Build history of the part. All positions in model axes, mm. A direction names the side the tool comes from. Coordinates: 2 decimals unless noted, no trailing zeros. Loops run counter-clockwise (first coordinate to the right, second up) from the corner with the lowest first, then second, coordinate; pieces in that order, holes last.
Item 1: Cut at A-A (y = -6). List the corners of the cut face in (x, z), and give its area (3 significant figures).
Item 2: Cut at D-D (x = -8.75). List the corners of the cut face in (y, z), and give its area (3 significant figures).
Item 3: Cut at C-C (x = 1.75). List the corners of the cut face in (y, z).
Item 4: Drill centre lines: line 1 along Y through (x, z) = (0, 15.8); line 2 along X through (y, z) = (8.5, 11); line 3 along Y through (x, z) = (6.75, 7.75). Where is each one in solid material? Low to high.
Item 5: Mould opens along X. For faces 1 (the face through (-3, -1, 11)), 2 (the face through (9.3, -11.8, 0.6)), 3 (the face through (-2.6, -12, 16.5)) say: released by +X, released by -X, zero draft, split by the parting line, or undercut.
Item 6: 3-axis set-ups, long thin cutter, end or side, ignore diameter. For faces 4 (the face through (1.01, -2.45, 8.26)), 5 (the face through (-10, 9.85, 6)): which of +Z, -Z, +X, -X, +Y, -Y reach the whole face in a straight line?
Item 7: Cut at B-B (z = 8). Count the separate pieces of the cut face and the enclosed holes in it, and give its area (3 significant figures).
Item 8: Flat gauge pins, fed straight in: pin 1 (0.7 mm diameter, centred on x = -1, y = -3.5, fed in from -Z); pin 2 (3 mm diameter, centred on x = 1, y = -1, fed in from -Z); pin 3 (3 mm diameter, centred on x = 1.5, y = 1, fed in from -Z). Where does each tip first touch, or does it go through?
Autodesk Inventor part; units mm, degrees
ref_plane "YZ Plane" through (0, 0, 0) normal (1, 0, 0) x (0, 1, 0)
ref_plane "XZ Plane" through (0, 0, 0) normal (0, 1, 0) x (-1, 0, 0)
ref_plane "XY Plane" through (0, 0, 0) normal (0, 0, 1) x (1, 0, 0)
sketch "スケッチ1" plane through (0, 0, 0) normal (0, 0, 1) x (1, 0, 0)
  circle A0 centre (0, 0) radius 5.1
  line L0 (10, -12.5) -> (-10, -12.5)
  line L1 (-10, -12.5) -> (-10, 12.5)
  line L2 (-10, 12.5) -> (10, 12.5)
  line L3 (10, 12.5) -> (10, -12.5)
  line L4 (10, -12.5) -> (-10, 12.5) construction
  line L5 (-10, -12.5) -> (10, 12.5) construction
  dimension "d0" = 10.2
  dimension "d1" = 25
  dimension "d2" = 20
extrude "押し出し1" add sketch "スケッチ1" along normal blind 17
sketch "スケッチ2" plane through (0, 0, 17) normal (0, 0, 1) x (1, 0, 0)
  circle A0 centre (0, 0) radius 5.1
extrude "押し出し2" add sketch "スケッチ2" against normal blind 12
sketch "スケッチ3" plane through (0, 0, 17) normal (0, 0, 1) x (1, 0, 0)
  point P0 (0, 0)
hole "穴1" at (0, 0, 17) direction (0, 0, -1) diameter 5.3 depth 58 counterbore diameter 11 counterbore depth 6
sketch "Sketch7" plane through (-10, -12.5, 0) normal (-1, 0, 0) x (0, 0, 1)
  line L0 (0, 25) -> (0, 0)
  line L1 (5, 7.4) -> (5, 17.6)
  line L2 (0, 17.6) -> (0, 7.4)
  point P0 (0, 12.5)
  point P1 (8, 6.5)
  point P2 (8, 18.5)
  dimension "d35" = 8
  dimension "d36" = 12
  dimension "d37" = 6
hole "Hole3" at (-10, -6, 8) at (-10, 6, 8) direction (1, 0, 0) diameter 4.5 depth 58
chamfer "Chamfer2" distance 3 angle 45 1 edges at (10, 0, 17)
sketch "Sketch8" plane through (-10, -12.5, 0) normal (-1, 0, 0) x (0, 0, 1)
  circle A0 centre (8, 6.5) radius 2.25
  circle A1 centre (8, 18.5) radius 2.25
  line L0 (0, 25) -> (0, 0)
  line L1 (0, 0) -> (17, 0)
  line L2 (17, 25) -> (17, 0)
  line L3 (0, 25) -> (17, 25)
  point P0 (0, 12.5)
extrude "Extrusion5" add sketch "Sketch8" along normal blind 5
sketch "Sketch9" plane through (0, 0, 17) normal (0, 0, 1) x (1, 0, 0)
  line L0 (7, 12.5) -> (7, -12.5)
  line L1 (7, 12.5) -> (-15, 12.5)
  line L2 (-15, -12.5) -> (-15, 12.5)
  line L3 (7, -12.5) -> (-15, -12.5)
  circle A0 centre (0, 0) radius 5.5
  line L4 (-15, 3.75) -> (-15, 8.25)
  line L5 (10, 8.25) -> (10, 3.75)
  line L6 (-15, -8.25) -> (-15, -3.75)
  line L7 (-15, -8.25) -> (-15, -3.75)
  line L8 (10, -3.75) -> (10, -8.25)
  line L9 (-10.9, 9.85) -> (-9.1, 9.85)
  line L10 (-9.1, 9.85) -> (-9.1, 2.15)
  line L11 (-9.1, 2.15) -> (-10.9, 2.15)
  line L12 (-10.9, 2.15) -> (-10.9, 9.85)
  line L13 (-10.9, 9.85) -> (-9.1, 2.15) construction
  line L14 (-9.1, 9.85) -> (-10.9, 2.15) construction
  line L15 (-10.9, -2.15) -> (-9.1, -2.15)
  line L16 (-9.1, -2.15) -> (-9.1, -9.85)
  line L17 (-9.1, -9.85) -> (-10.9, -9.85)
  line L18 (-10.9, -9.85) -> (-10.9, -2.15)
  line L19 (-10.9, -2.15) -> (-9.1, -9.85) construction
  line L20 (-9.1, -2.15) -> (-10.9, -9.85) construction
  line L21 (10, 8.25) -> (10, 3.75)
  point P0 (-10, 6)
  point P1 (-10, -6)
  point P2 (-10, 6)
  point P3 (-10, -6)
  point P4 (10, 6)
  point P5 (10, -6)
  point P6 (10, 6)
  dimension "d53" = 7.7
  dimension "d54" = 7.7
  dimension "d55" = 1.8
  dimension "d56" = 5
extrude "Extrusion6" cut sketch "Sketch9" against normal through all contours L9 L10 L11 L12 | L15 L16 L17 L18
sketch "Sketch10" plane through (0, 0, 17) normal (0, 0, 1) x (1, 0, 0)
  line L0 (-9.1, -2.15) -> (-9.1, -9.85)
  line L1 (-9.1, -9.85) -> (-10.9, -9.85)
  line L2 (-10.9, -9.85) -> (-10.9, -2.15)
  line L3 (-10.9, -2.15) -> (-9.1, -2.15)
  line L4 (-10.9, 9.85) -> (-9.1, 9.85)
  line L5 (-9.1, 9.85) -> (-9.1, 2.15)
  line L6 (-9.1, 2.15) -> (-10.9, 2.15)
  line L7 (-10.9, 2.15) -> (-10.9, 9.85)
  line L8 (7, 12.5) -> (7, -12.5)
  line L9 (7, 12.5) -> (-15, 12.5)
  line L10 (-15, -12.5) -> (-15, 12.5)
  line L11 (7, -12.5) -> (-15, -12.5)
  circle A0 centre (0, 0) radius 5.5
extrude "Extrusion7" add sketch "Sketch10" against normal blind 5 contours L0 L1 L2 L3 | L4 L5 L6 L7
chamfer "Chamfer4" distance 3 angle 45 1 edges at (-15, 0, 17)
chamfer "面取り7" distance 1 angle 45 14 edges at (-15, 12.5, 7) (-13.5, 12.5, 15.5) (-2.5, 12.5, 17) (8.5, 12.5, 15.5) (10, 12.5, 7) (10, -12.5, 7) (8.5, -12.5, 15.5) (-2.5, -12.5, 17) (-13.5, -12.5, 15.5) (-15, -12.5, 7) (-2.5, 12.5, 0) (-2.5, -12.5, 0) (10, 0, 0) (-15, 0, 0)
sketch "スケッチ11" plane through (0, 0, 5) normal (0, 0, -1) x (-1, 0, 0)
  circle A0 centre (0, 0) radius 2.65
  line L0 (2.65, 2.65) -> (-2.65, 2.65)
  line L1 (-2.65, 2.65) -> (-2.65, -2.65)
  line L2 (-2.65, -2.65) -> (2.65, -2.65)
  line L3 (2.65, -2.65) -> (2.65, 2.65)
  circle A1 centre (0, 0) radius 2.65
  line L4 (2.65, 2.65) -> (-2.65, -2.65) construction
  line L5 (-2.65, 2.65) -> (2.65, -2.65) construction
  point P0 (2.65, 0)
  point P1 (0, -2.65)
  point P2 (0, 2.65)
  point P3 (-2.65, 0)
extrude "押し出し8" cut sketch "スケッチ11" against normal blind 0.6 contours L3 L2 A0 | A0 L0 L3 | A0 L1 L0 | L2 L1 A0
sketch "スケッチ12" plane through (0, 0, 5) normal (0, 0, -1) x (-1, 0, 0)
  line L0 (-2.65, 2.65) -> (2.65, 2.65)
  line L1 (2.65, -2.65) -> (-2.65, -2.65)
  circle A0 centre (0, 0) radius 5.1
  line L2 (2.65, 5.3923) -> (-2.65, 5.3923)
  line L3 (-2.65, 5.3923) -> (-2.65, -5.3923)
  line L4 (-2.65, -5.3923) -> (2.65, -5.3923)
  line L5 (2.65, -5.3923) -> (2.65, 5.3923)
  line L6 (2.65, 5.3923) -> (-2.65, -5.3923) construction
  line L7 (-2.65, 5.3923) -> (2.65, -5.3923) construction
  point P0 (2.65, 2.65)
  point P1 (2.65, 4.3575)
  point P2 (-2.65, 4.3575)
  point P3 (2.65, -4.3575)
  point P4 (-2.65, -4.3575)
extrude "押し出し9" cut sketch "スケッチ12" against normal blind 0.3 contours L3 A0 L5 L0 | L1 L5 A0 L3
properties part number "Print_Parts_R" material "PC/ABS プラスチック"
Filled sheet:
1. outline: (-15, 1) - (-14, 0) - (-10.9, 0) - (-10.9, 5.75) - (-15, 5.75) - close; (-15, 10.25) - (-10.9, 10.25) - (-10.9, 12) - (-9.1, 12) - (-9.1, 10.25) - (10, 10.25) - (10, 14) - (7, 17) - (-12, 17) - (-15, 14) - close; (-9.1, 0) - (9, 0) - (10, 1) - (10, 5.75) - (-9.1, 5.75) - close
1. area: 289 mm2
2. outline: (-12.5, 1) - (-11.5, 0) - (11.5, 0) - (12.5, 1) - (12.5, 16) - (11.5, 17) - (-11.5, 17) - (-12.5, 16) - close; hole circle Ø4.5 at (-6, 8); hole circle Ø4.5 at (6, 8)
2. area: 391 mm2
3. outline: (-12.5, 1) - (-11.5, 0) - (-4.79, 0) - (-4.79, 5.3) - (-2.65, 5.3) - (-2.65, 5.6) - (-1.99, 5.6) - (-1.99, 11) - (-5.21, 11) - (-5.21, 17) - (-11.5, 17) - (-12.5, 16) - close; (1.99, 5.6) - (2.65, 5.6) - (2.65, 5.3) - (4.79, 5.3) - (4.79, 0) - (11.5, 0) - (12.5, 1) - (12.5, 16) - (11.5, 17) - (5.21, 17) - (5.21, 11) - (1.99, 11) - close; hole circle Ø4.5 at (-6, 8); hole circle Ø4.5 at (6, 8)
4. line 1: y = -12.5 to -5.5, 5.5 to 12.5
4. line 2: x = -15 to -10.9, -9.1 to 10
4. line 3: y = -12.5 to -8.24, -3.76 to 3.76, 8.24 to 12.5
5. face 1: undercut
5. face 2: released by +X
5. face 3: zero draft
6. face 4: +Z, -Z
6. face 5: -Z
7. separate pieces: 3
7. enclosed holes: 1
7. area: 364 mm2
8. pin 1: stops at z = 5.3
8. pin 2: stops at z = 5.6
8. pin 3: stops at z = 5
